For this review, take the finished solid that the model builds, in its own axes (mm). Face numbers are marked on the shaded views. A direction names the side the tool comes from. Coordinates: 2 decimals unless noted, no trailing zeros. Order: outer loops, then holes, each group sorted by start corner. A loop starts at its lowest first (then second) coordinate and runs counter-clockwise, first axis right, second up. Notation, with made-up numbers: (0.5, 53) -> (4.5, 53) arc R6 cw to (4.5, 60) -> close; hole circle Ø11 at (35.5, 63). An arc over 180 degrees is marked (long way). Answer as a JSON object with one key per item and string values. Group by question number.
1) Add section A-A, the plane y = 15.5. Write out the cut boundary in (x, z), then the cut area to 3 significant figures.
2) Add section D-D, the plane z = 47. Write out the cut boundary in (x, y), then the cut area to 3 significant figures.
3) Machinability: for the marked faces 1, 2 and 3, which of the approach directions +Z, -Z, +X, -X, +Y, -Y give a long, thin tool a straight path to every point of the face, cutting with its end or side? Answer none if there is none.
4) Wall thickness on L1, parallel to Y at x = 39, z = 39; L2, parallel to Z at x = 11, y = 91.5; L3, parallel to Y at x = 24, z = 32: over which ranges is each line inside the solid? List them lowest first.
5) Draft analysis for pull direction X (two halves, no side actions). For the marked faces 4, 5, 6 and 7, state which applies: +X half, -X half, draft (parallel to the pull), parting line (faces both ways), or undercut.
6) Add section B-B, the plane z = 39. Count the separate pieces of the cut face and the enclosed holes in it, then the cut area to 3 significant figures.
7) For pin 1 (12.5 mm diameter, centred on x = 19, y = 45.5, fed in from +Z); pin 2 (12 mm diameter, centred on y = 70, z = 33.5, fed in from -X); pin 3 (10 mm diameter, centred on x = 24, y = 84, fed in from -Z); pin 4 (5.5 mm diameter, centred on y = 101.5, z = 21, fed in from -X), all flat-tipped, find the tip position at first contact; note any pin that passes through.
8) Add section C-C, the plane y = 70. Write out the cut boundary in (x, z).
from build123d import *

# Parameters (mm, degrees)
BOSS_EXTRUDE1_DEPTH     = 80
SKETCH2_W               = 33
SKETCH2_H               = 110
CUT_EXTRUDE2_DEPTH      = 37.5
CUT_EXTRUDE6_DEPTH      = 55.5
SKETCH7_R               = 1.5000015
SKETCH7_R_2             = 1.499999754
SKETCH7_R_3             = 1.499999424
SKETCH7_R_4             = 1.499998917
CUT_EXTRUDE8_DEPTH      = 43
CUT_EXTRUDE8_DEPTH_BACK = 55.5
CUT_EXTRUDE9_DEPTH      = 110.5
CUT_EXTRUDE10_DEPTH     = 196.5
SKETCH11_R              = 2.10000039
SKETCH11_R_2            = 2.100000448
SKETCH11_R_3            = 2.1000011
SKETCH11_R_4            = 2.099999964
CUT_EXTRUDE11_DEPTH     = 196.5
CUT_EXTRUDE12_START     = 114.5
SKETCH12_R              = 15.500000658
CUT_EXTRUDE12_DEPTH     = 1
CUT_EXTRUDE13_START     = 114.5
SKETCH13_W              = 25
SKETCH13_H              = 6
CUT_EXTRUDE13_DEPTH     = 2


with BuildPart() as part:
    # Sketch1 → Boss-Extrude1 (new body)
    with BuildSketch(Plane.XY):
        Polygon((0, 114.5), (42, 114.5), (42, 0), (37.5, 0), (37.5, 18), (0, 92), align=None)
    extrude(amount=BOSS_EXTRUDE1_DEPTH)

    # Sketch2 → Cut-Extrude2 (cut)
    with BuildSketch(Plane(origin=(0, 0, 0), x_dir=(0, 0, -1), z_dir=(1, 0, 0))):
        with Locations((-39, 55)):
            Rectangle(SKETCH2_W, SKETCH2_H)
    extrude(amount=CUT_EXTRUDE2_DEPTH, mode=Mode.SUBTRACT)

    # Sketch6 → Cut-Extrude6 (cut)
    with BuildSketch(Plane(origin=(0, 0, 0), x_dir=(0, 0, -1), z_dir=(1, 0, 0))):
        Polygon((-17.5, 110), (-0.011922265, 110), (-0.011922265, 114.499832966), (14.004945748, 114.499832966), (14.004945748, 0), (-17.5, 0), align=None)
        Polygon((-60.5, 110), (-77.994888003, 110), (-77.985702515, 114.5), (-108.593167203, 114.5), (-108.593167203, 0), (-60.5, 0), align=None)
    extrude(amount=CUT_EXTRUDE6_DEPTH, mode=Mode.SUBTRACT)

    # Sketch7 → Cut-Extrude8 (cut, two sides)
    with BuildSketch(Plane(origin=(0, 0, 0), x_dir=(0, 0, -1), z_dir=(1, 0, 0))) as cut_extrude8_sk:
        with Locations((-39.000000948, 47.999997685)):
            Circle(SKETCH7_R)
        with Locations((-39, 35.499996297)):
            Circle(SKETCH7_R_2)
        with Locations((-39.000001283, 8.000001659)):
            Circle(SKETCH7_R_3)
        with Locations((-39.000000539, 15.500000933)):
            Circle(SKETCH7_R_4)
        with BuildLine():
            Line((-49.5, 106), (-28.187131882, 105.975372314))
            ThreePointArc((-28.187131882, 105.975372314), (-26.979186724, 105.298896246), (-26.5, 104))
            Line((-26.5, 104), (-26.5, 98))
            ThreePointArc((-26.5, 98), (-27.085785866, 96.585785866), (-28.5, 96))
            Line((-28.5, 96), (-49.5, 96))
            ThreePointArc((-49.5, 96), (-50.914215088, 96.585784912), (-51.5, 98))
            Line((-51.5, 98), (-51.5, 104))
            ThreePointArc((-51.5, 104), (-50.914215088, 105.414215088), (-49.5, 106))
        make_face()
    extrude(amount=CUT_EXTRUDE8_DEPTH, mode=Mode.SUBTRACT)
    extrude(cut_extrude8_sk.sketch, amount=-CUT_EXTRUDE8_DEPTH_BACK, mode=Mode.SUBTRACT)

    # Sketch8 → Cut-Extrude9 (cut)
    with BuildSketch(Plane.XY):
        with BuildLine():
            Line((33, 86), (13.022629738, 86))
            ThreePointArc((13.022629738, 86), (11.318500031, 85.046870918), (11.238623619, 83.095939636))
            Line((11.238623619, 83.095939636), (31.215991974, 43.673931122))
            ThreePointArc((31.215991974, 43.673931122), (33.464748466, 42.632740588), (35, 44.577987671))
            Line((35, 44.577987671), (35, 84))
            ThreePointArc((35, 84), (34.414214051, 85.414214051), (33, 86))
        make_face()
        with BuildLine():
            Line((9, 106), (33, 106))
            ThreePointArc((33, 106), (34.414214051, 105.414214051), (35, 104))
            Line((35, 104), (35, 98))
            ThreePointArc((35, 98), (34.414214051, 96.585785949), (33, 96))
            Line((33, 96), (9, 96))
            ThreePointArc((9, 96), (7.585785856, 96.585786135), (6.999999046, 98))
            Line((6.999999046, 98), (6.999999046, 104))
            ThreePointArc((6.999999046, 104), (7.585785772, 105.414213949), (9, 106))
        make_face()
    extrude(amount=CUT_EXTRUDE9_DEPTH, mode=Mode.SUBTRACT)

    # Sketch10 → Cut-Extrude10 (cut)
    with BuildSketch(Plane(origin=(0, 0, 0), x_dir=(1, 0, 0), z_dir=(0, 1, 0))):
        with BuildLine():
            Line((0, -6.136648178), (0, 15.4695464))
            Line((0, 15.4695464), (11.339564335, 15.4695464))
            Line((11.339564335, 15.4695464), (42, 15.4695464))
            Line((42, 15.4695464), (42, -6.136648178))
            ThreePointArc((42, -6.136648178), (21, -2.155e-06), (0, -6.136648178))
        make_face()
        with BuildLine():
            Line((0, -71.863349915), (0, -99.275377961))
            Line((0, -99.275377961), (42, -99.275377961))
            Line((42, -99.275377961), (42, -71.863349915))
            ThreePointArc((42, -71.863349915), (21, -78.000003087), (0, -71.863349915))
        make_face()
    extrude(amount=CUT_EXTRUDE10_DEPTH, mode=Mode.SUBTRACT)

    # Sketch11 → Cut-Extrude11 (cut)
    with BuildSketch(Plane(origin=(0, 0, 0), x_dir=(1, 0, 0), z_dir=(0, 1, 0))):
        with Locations((10.570675656, -6.901843556)):
            Circle(SKETCH11_R)
        with Locations((31.429323256, -6.901843615)):
            Circle(SKETCH11_R_2)
        with Locations((31.429323915, -71.098157164)):
            Circle(SKETCH11_R_3)
        with Locations((10.570676027, -71.098155911)):
            Circle(SKETCH11_R_4)
    extrude(amount=CUT_EXTRUDE11_DEPTH, mode=Mode.SUBTRACT)

    # Sketch12 → Cut-Extrude12 (cut)
    with BuildSketch(Plane(origin=(0, 0, 0), x_dir=(1, 0, 0), z_dir=(0, 1, 0)).offset(CUT_EXTRUDE12_START)):
        with Locations((20.999998985, -39.000002134)):
            Circle(SKETCH12_R)
    extrude(amount=-CUT_EXTRUDE12_DEPTH, mode=Mode.SUBTRACT)

    # Sketch13 → Cut-Extrude13 (cut)
    with BuildSketch(Plane(origin=(0, 0, 0), x_dir=(1, 0, 0), z_dir=(0, 1, 0)).offset(CUT_EXTRUDE13_START)):
        with Locations((29.5, -39)):
            Rectangle(SKETCH13_W, SKETCH13_H)
    extrude(amount=-CUT_EXTRUDE13_DEPTH, mode=Mode.SUBTRACT)


solid = part.part
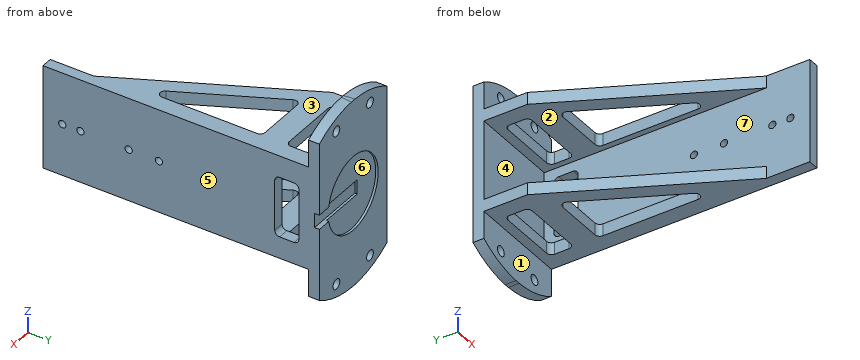
Output values:
{
 "1": {"outline": "(37.5, 17.5) -> (42, 17.5) -> (42, 37.5) -> (37.5, 37.5) -> close; (37.5, 40.5) -> (42, 40.5) -> (42, 60.5) -> (37.5, 60.5) -> close", "area": "180 mm²"},
 "2": {"outline": "(0, 110) -> (37.5, 110) -> (37.5, 106) -> (42, 106) -> (42, 114.5) -> (34.28, 114.5) -> (34.28, 113.5) -> (7.72, 113.5) -> (7.72, 114.5) -> (0, 114.5) -> close; (37.5, 0) -> (42, 0) -> (42, 96) -> (37.5, 96) -> close", "area": "612 mm²"},
 "3": {"face 1": "-Z, +X, -X, -Y", "face 2": "-X, -Y", "face 3": "+Z, +X, -X, -Y"},
 "4": {"L1": "y = 0 to 6.5, 9.5 to 14, 17 to 34, 37 to 46.5, 49.5 to 96, 105.99 to 112.5", "L2": "z = 17.5 to 22.5, 55.5 to 60.5", "L3": "y = 110 to 113.5"},
 "5": {"face 4": "draft", "face 5": "+X half", "face 6": "undercut", "face 7": "-X half"},
 "6": {"separate pieces": "6", "enclosed holes": "0", "area": "524 mm²"},
 "7": {"pin 1": "stops at z = 60.5", "pin 2": "stops at x = 37.5", "pin 3": "stops at z = 17.5", "pin 4": "stops at x = 0"},
 "8": {"outline": "(11.15, 17.5) -> (17.88, 17.5) -> (17.88, 22.5) -> (11.15, 22.5) -> close; (11.15, 55.5) -> (17.88, 55.5) -> (17.88, 60.5) -> (11.15, 60.5) -> close; (35, 17.5) -> (42, 17.5) -> (42, 60.5) -> (35, 60.5) -> (35, 55.5) -> (37.5, 55.5) -> (37.5, 22.5) -> (35, 22.5) -> close"}
}
